Geometry check sheet. Reference: the model listing, model coordinates, mm. A direction names the side the tool comes from. Round coordinates to 2 decimals unless told otherwise and drop trailing zeros. Write each loop counter-clockwise with the first axis right and the second up, starting at its lowest first coordinate (ties: lowest second). Pieces come first, ordered by that corner, then holes. Notation, with made-up numbers: M 6.25,85 L 46.25,85 A6 ccw 46.25,96 Z; hole C 77.5,88 d2. An arc over 180 degrees is marked long. Use a Markdown table: item, result.
```python
from build123d import *

# Parameters (mm, degrees)
SKETCH1_W           = 660
SKETCH1_H           = 80
BOSS_EXTRUDE1_DEPTH = 80
BOSS_EXTRUDE2_START = 320
SKETCH2_W           = 100
SKETCH2_H           = 100
BOSS_EXTRUDE2_DEPTH = 10
BOSS_EXTRUDE3_START = -280
SKETCH2_2_W         = 100
SKETCH2_2_H         = 100
BOSS_EXTRUDE3_DEPTH = 10
BOSS_EXTRUDE4_START = -290
SKETCH2_4_W         = 80
SKETCH2_4_H         = 80
BOSS_EXTRUDE4_DEPTH = 100
SKETCH4_R           = 12.5
BOSS_EXTRUDE5_DEPTH = 80
CUT_EXTRUDE1_DEPTH  = 80


with BuildPart() as part:
    # Sketch1 → Boss-Extrude1 (new body)
    with BuildSketch(Plane(origin=(0, 0, 0), x_dir=(1, 0, 0), z_dir=(0, 1, 0))):
        Rectangle(SKETCH1_W, SKETCH1_H)
    extrude(amount=BOSS_EXTRUDE1_DEPTH)

    # Sketch2 → Boss-Extrude2 (add)
    with BuildSketch(Plane(origin=(0, 0, 0), x_dir=(0, 0, -1), z_dir=(1, 0, 0)).offset(BOSS_EXTRUDE2_START)):
        with Locations((0, 40)):
            Rectangle(SKETCH2_W, SKETCH2_H)
    extrude(amount=BOSS_EXTRUDE2_DEPTH)

    # Sketch2<2> → Boss-Extrude3 (add)
    with BuildSketch(Plane(origin=(0, 0, 0), x_dir=(0, 0, -1), z_dir=(1, 0, 0)).offset(BOSS_EXTRUDE3_START)):
        with Locations((0, 40)):
            Rectangle(SKETCH2_2_W, SKETCH2_2_H)
    extrude(amount=-BOSS_EXTRUDE3_DEPTH)

    # Sketch2<4> → Boss-Extrude4 (add)
    with BuildSketch(Plane(origin=(0, 0, 0), x_dir=(0, 0, -1), z_dir=(1, 0, 0)).offset(BOSS_EXTRUDE4_START)):
        with Locations((0, 40)):
            Rectangle(SKETCH2_4_W, SKETCH2_4_H)
    extrude(amount=-BOSS_EXTRUDE4_DEPTH)

    # Sketch4 → Boss-Extrude5 (add)
    with BuildSketch(Plane.XY.offset(40)):
        with BuildLine():
            Line((-430, 0), (-390, 0))
            Line((-390, 0), (-390, 80))
            Line((-390, 80), (-430, 80))
            ThreePointArc((-430, 80), (-470, 40), (-430, 0))
        make_face()
        with Locations((-430, 40)):
            Circle(SKETCH4_R, mode=Mode.SUBTRACT)
    extrude(amount=-BOSS_EXTRUDE5_DEPTH)

    # Sketch5 → Cut-Extrude1 (cut)
    with BuildSketch(Plane(origin=(0, 80, 0), x_dir=(1, 0, 0), z_dir=(0, 1, 0))):
        with BuildLine():
            Line((-470, 20), (-430, 20))
            Line((-430, 20), (-410, 20))
            ThreePointArc((-410, 20), (-390, 0), (-410, -20))
            Line((-410, -20), (-430, -20))
            Line((-430, -20), (-470, -20))
            Line((-470, -20), (-470, 20))
        make_face()
    extrude(amount=-CUT_EXTRUDE1_DEPTH, mode=Mode.SUBTRACT)


solid = part.part
```
Item 1: Material ranges on line 1 along Y through (x, z) = (-430, -25.25); line 2 along Z through (x, y) = (-413.5, 47); line 3 along Y through (x, z) = (44, 19), recorded low to high. Write a range as from..to.
Outcome:
| item | result |
|---|---|
| line 1 | y = 0..27.5, 52.5..80 |
| line 2 | z = -40..-20, 20..40 |
| line 3 | y = 0..80 |
Item 2: Access from +Z, -Z, +X, -X, +Y, -Y to the whole of each face (thin tool, end or side, straight path). Record for faces 1 (the face through (-381, 41, -40)), 2 (the face through (-440, 49, -20)), 3 (the face through (320, 41, 45)), 4 (the face through (-290, 41, 45)), 5 (the face through (16, 80, -1)).
Outcome:
| item | result |
|---|---|
| face 1 | -Z, -X, +Y, -Y |
| face 2 | -X, +Y, -Y |
| face 3 | none |
| face 4 | -X |
| face 5 | +Z, -Z, +Y |
Item 3: Cross-section at A-A, the plane y = 40. Record the cut outline in (x, z).
Outcome:
| item | result |
|---|---|
| outline | M -470,-40 L -442.5,-40 L -442.5,-20 L -470,-20 Z; M -470,20 L -442.5,20 L -442.5,40 L -470,40 Z; M -417.5,-40 L -290,-40 L -290,-50 L -280,-50 L -280,-40 L 320,-40 L 320,-50 L 330,-50 L 330,50 L 320,50 L 320,40 L -280,40 L -280,50 L -290,50 L -290,40 L -417.5,40 L -417.5,20 L -410,20 A20 cw -410,-20 L -417.5,-20 Z |
Item 4: Cross-section at C-C, the plane x = -154.5. Record the cut outline in (y, z), and give its area (3 significant figures).
Outcome:
| item | result |
|---|---|
| outline | M 0,-40 L 80,-40 L 80,40 L 0,40 Z |
| area | 6,400 mm2 |
Item 5: Cross-section at B-B, the plane z = -12. Record the cut outline in (x, y), and give its area (3 significant figures).
Outcome:
| item | result |
|---|---|
| outline | M -394,0 L -290,0 L -290,-10 L -280,-10 L -280,0 L 320,0 L 320,-10 L 330,-10 L 330,90 L 320,90 L 320,80 L -280,80 L -280,90 L -290,90 L -290,80 L -394,80 Z |
| area | 58,300 mm2 |
Item 6: Go/stop test with flat-tipped pins: pin 1 (24 mm diameter, centred on x = -363, z = 8.5, fed in from -Y); pin 2 (10 mm diameter, centred on x = -259.5, z = 38, fed in from +Y); pin 3 (8 mm diameter, centred on x = 171, y = 32.5, fed in from -Z). Record where each tip stops, or that it passes through.
Outcome:
| item | result |
|---|---|
| pin 1 | stops at y = 0 |
| pin 2 | stops at y = 80 |
| pin 3 | stops at z = -40 |
Item 7: Mould release check, pull along X, two halves, no side actions. Record for faces 6 (the face through (16, 0, -1)), 7 (the face through (-343, 80, 1)), 8 (the face through (330, 41, 1)): +X half, -X half, draft (parallel to the pull), parting line (faces both ways), or undercut.
Outcome:
| item | result |
|---|---|
| face 6 | undercut |
| face 7 | draft |
| face 8 | +X half |
